Could you check a few things on this model? Use its own coordinates, in mm. A direction names the side the tool comes from. Give positions to 0.01 mm unless a question says otherwise; leave off trailing zeros. Loops run counter-clockwise (first coordinate to the right, second up) from the corner with the lowest first, then second, coordinate; pieces in that order, holes last. Notation, with made-up numbers: M 6.5,68.5 L 42.5,68.5 A15 ccw 42.5,96.5 Z; hole C 81.25,12 d5. An arc over 180 degrees is marked long. Use a Markdown table: item, result. Add a question column.
1) We'd pull the mould along X, two halves only. Please class faces 1 (the flat face through (10, -14.679, 3)), 2 (the flat face through (-2.468, -38, 5)), 3 (the flat face through (2.412, -38, 5)): +X half, -X half, draft (parallel to the pull), parting line (faces both ways), or undercut.
2) Suppose I cut it at C-C on x = 0. List the corners of the cut face in (y, z) for me.
3) Suppose I cut it at B-B on y = -13. List the corners of the cut face in (x, z) for me, and give its area (3 significant figures).
4) Suppose I cut it at A-A on z = 3. List the corners of the cut face in (x, y) for me, and give its area (3 significant figures).
5) If I drill on line 1 along Y through (x, z) = (0, 29); line 2 along Z through (x, y) = (6, -17), over which ranges is the centre line in solid material (lowest first)? Write a range as [from, to].
6) Suppose I cut it at D-D on y = 0. List the corners of the cut face in (x, z) for me.
7) Will these pins go through, and if not, where does the flat tip stop? pin 1 Ø8 at (x, z) = (13, 32) entering from -Y; pin 2 Ø7 at (y, z) = (-33.5, 13) entering from +X; pin 3 Ø8 at (x, y) = (10, -7) entering from -Z.
8) Which directions (+Z, -Z, +X, -X, +Y, -Y) give clear straight access to the entire face, cutting with the end or side of a thin tool? Please do faces 4 (the flat face through (13.268, -13, 3)), 5 (the flat face through (0, -27.48, -2)), 6 (the cylindrical face through (-2.994, 22.804, 33.129)), 7 (the flat face through (0, -36.941, 11)), 8 (the flat face through (0, -39, 21.13)).
```python
from build123d import *

# Parameters (mm, degrees)
F0_R     = 30
F1_DEPTH = 60
F2_T     = -7
F3_W     = 6
F3_H     = 4
F4_DEPTH = 7
F6_DEPTH = 5
F7_W     = 4.8802027013
F7_H     = 21.1299806833
F7_H_2   = 5
F8_DEPTH = 5


with BuildPart() as f1:
    # F0 (on Top) → F1 (new body)
    with BuildSketch(Plane.XY):
        Circle(F0_R)
    extrude(amount=F1_DEPTH)

    # F2
    f2_openings = [f1.faces().sort_by_distance(p)[0] for p in [
        (0, 0, 60),
    ]]
    offset(amount=F2_T, openings=f2_openings)

    # F3 (on face) → F4 (cut)
    with BuildSketch(Plane(origin=(0, 0, 0), x_dir=(1, 0, 0), z_dir=(0, 0, -1))):
        with Locations((10.2678574622, 12.6785714924)):
            Rectangle(F3_W, F3_H)
    extrude(amount=-F4_DEPTH, mode=Mode.SUBTRACT)

    # F5 (on face) → F6 (join)
    with BuildSketch(Plane(origin=(0, 0, 0), x_dir=(1, 0, 0), z_dir=(0, 0, -1))):
        with BuildLine():
            Line((-2.4681275245, 36.9405262172), (-2.4681275245, 29.8983000608))
            ThreePointArc((-2.4681275245, 29.8983000608), (-0.0281193423, 29.9999868217), (2.4120751768, 29.9028743324))
            Line((2.4120751768, 29.9028743324), (2.4120751768, 36.9405262172))
            Line((2.4120751768, 36.9405262172), (-2.4681275245, 36.9405262172))
        make_face()
        with BuildLine():
            Line((-2.4681275245, 29.8983000608), (-2.4681275245, 27.4804420769))
            Line((-2.4681275245, 27.4804420769), (2.4120751768, 27.4804420769))
            Line((2.4120751768, 27.4804420769), (2.4120751768, 29.9028743324))
            ThreePointArc((2.4120751768, 29.9028743324), (-0.0281193423, 29.9999868217), (-2.4681275245, 29.8983000608))
        make_face()
    extrude(amount=F6_DEPTH)

    # F7 (on face) → F8 (join)
    with BuildSketch(Plane.XZ.offset(36.9405262172)):
        with Locations((-0.0280261738, 10.5649903417)):
            Rectangle(F7_W, F7_H)
        with Locations((-0.0280261738, -2.5)):
            Rectangle(F7_W, F7_H_2)
    extrude(amount=F8_DEPTH)


solid = f1.part
```
Answer block:
| question | item | result |
|---|---|---|
| 1 | face 1 | undercut |
| 1 | face 2 | -X half |
| 1 | face 3 | +X half |
| 2 | outline | M -41.94,-5 L -27.48,-5 L -27.48,0 L 30,0 L 30,60 L 23,60 L 23,7 L -23,7 L -23,60 L -30,60 L -30,0 L -36.94,0 L -36.94,21.13 L -41.94,21.13 Z |
| 3 | outline | M -27.04,0 L 7.27,0 L 7.27,7 L -18.97,7 L -18.97,60 L -27.04,60 Z; M 13.27,0 L 27.04,0 L 27.04,60 L 18.97,60 L 18.97,7 L 13.27,7 Z |
| 3 | area | 1,190 mm^2 |
| 4 | outline | C 0,0 d60; M -2.47,-41.94 L 2.41,-41.94 L 2.41,-36.94 L -2.47,-36.94 Z; hole M 7.27,-14.68 L 13.27,-14.68 L 13.27,-10.68 L 7.27,-10.68 Z |
| 4 | area | 2,830 mm^2 |
| 5 | line 1 | y = [-30, -23], [23, 30] |
| 5 | line 2 | z = [0, 7] |
| 6 | outline | M -30,0 L 30,0 L 30,60 L 23,60 L 23,7 L -23,7 L -23,60 L -30,60 Z |
| 7 | pin 1 | stops at y = -28.62 |
| 7 | pin 2 | stops at x = 2.41 |
| 7 | pin 3 | stops at z = 0 |
| 8 | face 4 | +Z, -Z |
| 8 | face 5 | -Z, +X, -X, +Y |
| 8 | face 6 | +Z |
| 8 | face 7 | +Z, +X, -X |
| 8 | face 8 | +Z, +X, -X, -Y |
